Answer from the drawing. Dimensions are ordinates in mm from the lowest x, y and z of the part. A direction names the side the tool comes from. Give positions to 0.01 mm unless a question says otherwise; leave off trailing zeros. Loops run counter-clockwise (first coordinate to the right, second up) from the corner with the lowest first, then second, coordinate; pieces in that order, holes last. Notation, with made-up numbers: (56.5, 51.5) - (114.5, 51.5) arc R13 cw to (114.5, 61.5) - close; hole circle Ø4 at (14, 83). An arc over 180 degrees is marked (long way). One line per question, with ' | ' between items. Start each with the question number.
1. Each of these flat-tipped pins is pushed along its axis until it touches: pin 1 (1.5 mm diameter, centred on x = 20.41, y = 51.44, fed in from -Z); pin 2 (1.5 mm diameter, centred on x = 36.5, z = 5, fed in from -Y); pin 3 (1 mm diameter, centred on x = 51, z = 5.5, fed in from -Y); pin 4 (1 mm diameter, centred on x = 24, z = 11, fed in from -Y). Where does it stop, or does it pass through?
2. Section D-D (x = 41.5) is taken. Determine the outline of the cut face in (y, z), plus the area to 3 significant figures.
3. Section A-A (x = 29.5) is taken. Determine the outline of the cut face in (y, z).
4. Find the intervals of material crossed by line 1 (Y direction, x = 29.5, z = 6.25); line 2 (X direction, y = 30, z = 8) (1 decimal); line 3 (Y direction, x = 20, z = 11), in increasing order.
5. Which of the six approach directions +Z, -Z, +X, -X, +Y, -Y give full straight-line access (tool end or side, diameter ignored) to the marked faces 1 and 2?
6. Section B-B (z = 3.75) is taken. Give the number of separate pieces and of enclosed holes in the cut face, plus the area to 3 significant figures.
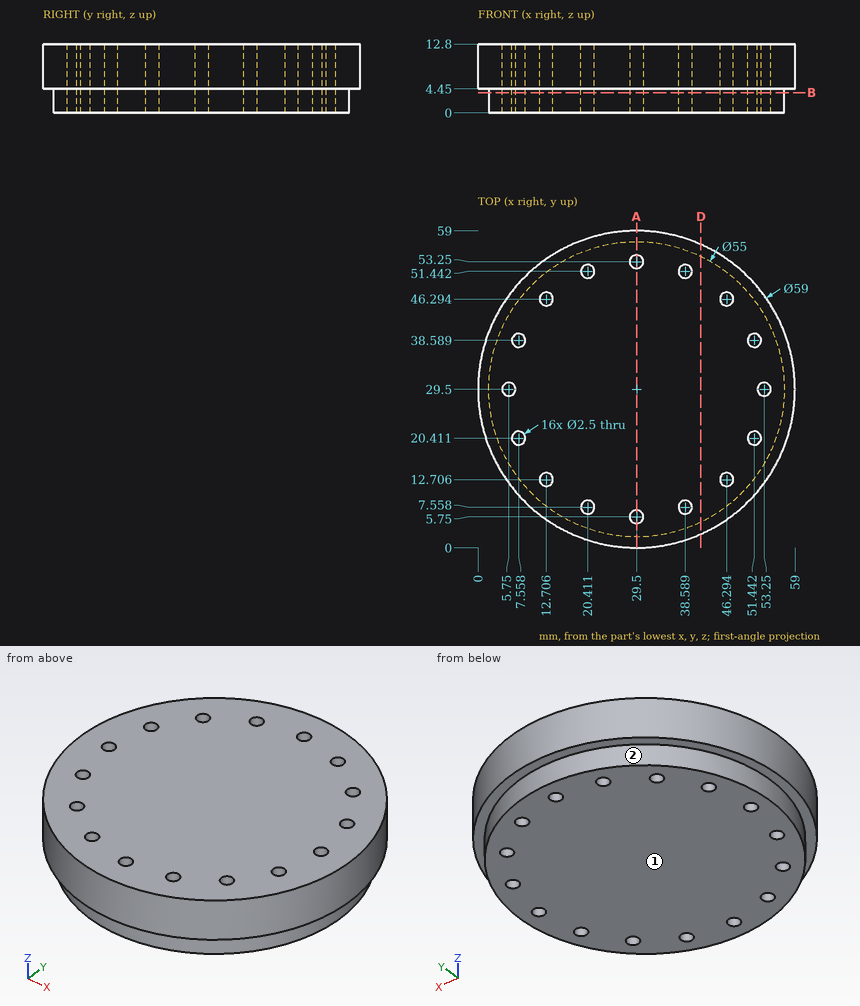
Conclusion:
1) pin 1: through | pin 2: y = 0.67 | pin 3: y = 8.78 | pin 4: y = 0.43
2) outline: (2.55, 4.45) - (4.76, 4.45) - (4.76, 0) - (54.24, 0) - (54.24, 4.45) - (56.45, 4.45) - (56.45, 12.8) - (2.55, 12.8) - close | area: 670 mm²
3) outline: (0, 4.45) - (2, 4.45) - (2, 0) - (4.5, 0) - (4.5, 12.8) - (0, 12.8) - close; (7, 0) - (52, 0) - (52, 12.8) - (7, 12.8) - close; (54.5, 0) - (57, 0) - (57, 4.45) - (59, 4.45) - (59, 12.8) - (54.5, 12.8) - close
4) line 1: 0 to 4.5, 7 to 52, 54.5 to 59 | line 2: 0 to 4.6, 6.9 to 52.1, 54.4 to 59 | line 3: 1.57 to 6.38, 8.74 to 50.26, 52.62 to 57.43
5) face 1: -Z, +X, -X, +Y, -Y | face 2: -Z
6) separate pieces: 1 | enclosed holes: 16 | area: 2,300 mm²
